from build123d import *

# Parameters (mm, degrees)
EXTRUDE_START       = -0.0001
EXTRUDE_2_OUTLINE_R = 2.2
EXTRUDE_2_DEPTH     = 5.0001
SKETCH_3_R          = 3.5
SKETCH_3_R_2        = 2.2
CUT_EXTRUDE_1_DEPTH = 2
CHAMFER_1_SIZE      = 0.5


# Read off the part's stored shape, not the designer's step: 凸台-拉伸2
with BuildPart() as part:
    # 凸台-拉伸2 outline → 凸台-拉伸2 (new body)
    with BuildSketch(Plane(origin=(0, 0, 0), x_dir=(1, 0, 0), z_dir=(0, 1, 0)).offset(EXTRUDE_START)):
        with BuildLine():
            Line((47, 5), (0, 5))
            ThreePointArc((0, 5), (-5, 0), (0, -5))
            Line((0, -5), (47, -5))
            ThreePointArc((47, -5), (52, 0), (47, 5))
        make_face()
        Circle(EXTRUDE_2_OUTLINE_R, mode=Mode.SUBTRACT)
        with Locations((47, 0)):
            Circle(EXTRUDE_2_OUTLINE_R, mode=Mode.SUBTRACT)
    extrude(amount=EXTRUDE_2_DEPTH)

    # 草图3 → 切除-拉伸1 (cut)
    with BuildSketch(Plane.XZ.offset(0.0001)):
        with Locations(Location((47, 0, 0), (0, 0, 270))):
            Circle(SKETCH_3_R)
        with Locations(Location((47, 0, 0), (0, 0, 90))):
            Circle(SKETCH_3_R_2, mode=Mode.SUBTRACT)
    extrude(amount=-CUT_EXTRUDE_1_DEPTH, mode=Mode.SUBTRACT)

    # 倒角1
    chamfer_1_edges = [part.edges().sort_by_distance(p)[0] for p in [
        (52, -0.0001, 0),
        (23.5, -0.0001, -5),
        (-5, 5, 0),
        (23.5, 5, 5),
        (52, 5, 0),
        (23.5, 5, -5),
        (47, -0.0001, 3.5),
        (-5, -0.0001, 0),
        (23.5, -0.0001, 5),
    ]]
    chamfer(chamfer_1_edges, length=CHAMFER_1_SIZE)


solid = part.part
Input: part model. Units: mm. Frame: model coordinates. A direction names the side the tool comes from. Coordinates: 2 decimals unless noted, no trailing zeros. Loops run counter-clockwise (first coordinate to the right, second up) from the corner with the lowest first, then second, coordinate; pieces in that order, holes last. Notation, with made-up numbers: (-39, -19) - (-16, -19) arc R9 cw to (-16, -15) - close; hole circle Ø1 at (4.5, 53). An arc over 180 degrees is marked (long way). Answer in a Markdown table with one row per item. Add a question column.
Item 1: Line query: line 1 along X through (y, z) = (1.4, 0); line 2 along X through (y, z) = (4.3, 0); line 3 along Z through (x, y) = (47, 2.9). Output: solid intervals per line, ascending. Write a range as [from, to].
Item 2: Mould query, pull axis Z, two halves, no side actions, for faces 1 (the cylindrical face through (50.47, 1.24, 0.46)), 2 (the flat face through (23, 0, 0)), 3 (the conical face through (51.64, 4.86, 0.1)). Classes: released by +Z, released by -Z, zero draft, split by the parting line, or undercut.
Item 3: Contact query for flat-ended pins moving along their axis: P1, Ø1.5, axis at y = 1, z = 3.5, coming from the -X side; P2, Ø3, axis at y = 4, z = 2.5, coming from the -X side. Output: stop coordinate, or through.
Item 4: Section query B-B on y = 3.75. Return the cut outline in (x, z), then the cut area to 3 significant figures.
Item 5: Section query A-A on z = 0. Return the cut outline in (x, y).
Item 6: Access query for faces 4 (the cylindrical face through (2.1, 2.46, -0.66)), 5 (the flat face through (45, 2, 2)). Directions: +Z, -Z, +X, -X, +Y, -Y. A direction counts if a zero-diameter tool reaches every point of the face in a straight line with its end or side. Return the directions, or none.
Recorded:
| question | item | result |
|---|---|---|
| 1 | line 1 | [-5, -2.2], [2.2, 43.5], [50.5, 52] |
| 1 | line 2 | [-5, -2.2], [2.2, 44.8], [49.2, 52] |
| 1 | line 3 | [-5, -2.2], [2.2, 5] |
| 2 | face 1 | undercut |
| 2 | face 2 | zero draft |
| 2 | face 3 | split by the parting line |
| 3 | P1 | x = -4.18 |
| 3 | P2 | x = -4.9 |
| 4 | outline | (0, -5) - (47, -5) arc R5 ccw to (47, 5) - (0, 5) arc R5 ccw to start; hole circle Ø4.4 at (0, 0); hole circle Ø4.4 at (47, 0) |
| 4 | area | 518 mm^2 |
| 5 | outline | (-5, 0.5) - (-4.5, 0) - (-2.2, 0) - (-2.2, 5) - (-4.5, 5) - (-5, 4.5) - close; (2.2, 0) - (43, 0) - (43.5, 0.5) - (43.5, 2) - (44.8, 2) - (44.8, 5) - (2.2, 5) - close; (49.2, 2) - (50.5, 2) - (50.5, 0.5) - (51, 0) - (51.5, 0) - (52, 0.5) - (52, 4.5) - (51.5, 5) - (49.2, 5) - close |
| 6 | face 4 | +Y, -Y |
| 6 | face 5 | -Y |
